Geometry check sheet. Reference: the model listing, model coordinates, mm. Face numbers are marked on the shaded views. A direction names the side the tool comes from. Coordinates: 2 decimals unless noted, no trailing zeros. Order: outer loops, then holes, each group sorted by start corner. A loop starts at its lowest first (then second) coordinate and runs counter-clockwise, first axis right, second up. Notation, with made-up numbers: (65, 19) - (86, 19) arc R12 cw to (86, 23) - close; hole circle Ø4 at (73, 37). An arc over 180 degrees is marked (long way). Put each result on its own line as item: value.
from build123d import *

# Parameters (mm, degrees)
SKETCH1_W           = 39.7
SKETCH1_H           = 39.7
BOSS_EXTRUDE1_DEPTH = 1
BOSS_EXTRUDE2_DEPTH = 13.6
SHELL1_START        = -12.6
SHELL1_DEPTH        = 13.6
SKETCH3_W           = 39.7
SKETCH3_H           = 39.7
SKETCH3_W_2         = 38.7
SKETCH3_H_2         = 38.7
CUT_EXTRUDE1_DEPTH  = 0.5
CUT_EXTRUDE2_REACH  = 33.642
SKETCH4_W           = 2
SKETCH4_H           = 0.3


# Read off the part's stored shape, not the designer's step: Shell1
with BuildPart() as part:
    # Sketch1 → Boss-Extrude1 (new body)
    with BuildSketch(Plane.XY):
        Rectangle(SKETCH1_W, SKETCH1_H)
    extrude(amount=BOSS_EXTRUDE1_DEPTH)

    # Sketch2 → Boss-Extrude2 (add)
    with BuildSketch(Plane(origin=(0, 0, 0), x_dir=(-1, 0, 0), z_dir=(0, 0, -1))):
        with BuildLine():
            Line((-8.3, -17.85), (8.3, -17.85))
            Line((8.3, -17.85), (8.3, -5.272366093))
            ThreePointArc((8.3, -5.272366093), (0, -0.85), (-8.3, -5.272366093))
            Line((-8.3, -5.272366093), (-8.3, -17.85))
        make_face()
    extrude(amount=BOSS_EXTRUDE2_DEPTH)

    # Shell1 outline → Shell1 (cut)
    with BuildSketch(Plane.XY.offset(SHELL1_START)):
        with BuildLine():
            Line((7.3, -16.85), (7.3, -5.585971125))
            ThreePointArc((7.3, -5.585971125), (0, -1.85), (-7.3, -5.585971125))
            Line((-7.3, -5.585971125), (-7.3, -16.85))
            Line((-7.3, -16.85), (7.3, -16.85))
        make_face()
    extrude(amount=SHELL1_DEPTH, mode=Mode.SUBTRACT)

    # Sketch3 → Cut-Extrude1 (cut)
    with BuildSketch(Plane.XY.offset(1)):
        Rectangle(SKETCH3_W, SKETCH3_H)
        Rectangle(SKETCH3_W_2, SKETCH3_H_2, mode=Mode.SUBTRACT)
    extrude(amount=-CUT_EXTRUDE1_DEPTH, mode=Mode.SUBTRACT)

    # Sketch4 → Cut-Extrude2 (cut, up to next)
    with BuildSketch(Plane(origin=(0, 0, -13.6), x_dir=(-1, 0, 0), z_dir=(0, 0, -1)), mode=Mode.PRIVATE) as cut_extrude2_sk1:
        with Locations((-5.5, -15.7)):
            Rectangle(SKETCH4_W, SKETCH4_H)
    cut_extrude2_tool1 = extrude(cut_extrude2_sk1.sketch, amount=-CUT_EXTRUDE2_REACH, mode=Mode.PRIVATE) & part.part
    # Sketch4 → Cut-Extrude2 (cut, up to next)
    with BuildSketch(Plane(origin=(0, 0, -13.6), x_dir=(-1, 0, 0), z_dir=(0, 0, -1)), mode=Mode.PRIVATE) as cut_extrude2_sk2:
        with Locations((5.5, -15.7)):
            Rectangle(SKETCH4_W, SKETCH4_H)
    cut_extrude2_tool2 = extrude(cut_extrude2_sk2.sketch, amount=-CUT_EXTRUDE2_REACH, mode=Mode.PRIVATE) & part.part
    add(cut_extrude2_tool1.solids().sort_by_distance((5.5, -15.7, -13.6))[0], mode=Mode.SUBTRACT)
    add(cut_extrude2_tool2.solids().sort_by_distance((-5.5, -15.7, -13.6))[0], mode=Mode.SUBTRACT)


solid = part.part
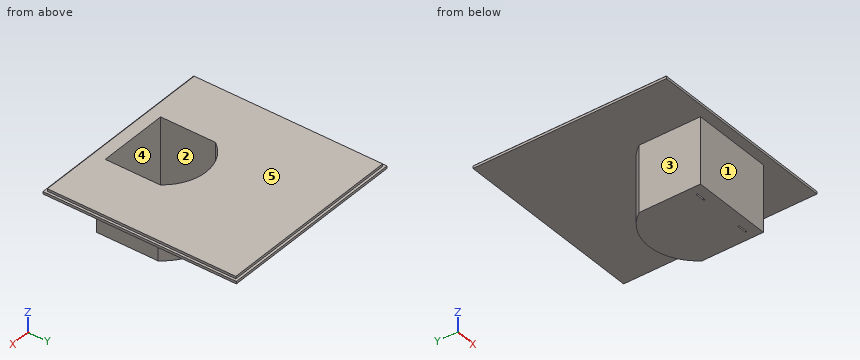
Q1. Section check A-A on z = -4.25. Record the boundary of the cut face in (x, y).
Answer block:
outline: (-8.3, -17.85) - (8.3, -17.85) - (8.3, -5.27) arc R10 ccw to (-8.3, -5.27) - close; hole (-7.3, -16.85) - (7.3, -16.85) - (7.3, -5.59) arc R9 ccw to (-7.3, -5.59) - close
Q2. Section check D-D on y = -4. Record the boundary of the cut face in (x, z).
Answer block:
outline: (-19.85, 0) - (-7.29, 0) - (-7.29, -13.6) - (7.29, -13.6) - (7.29, 0) - (19.85, 0) - (19.85, 0.5) - (19.35, 0.5) - (19.35, 1) - (5.84, 1) - (5.84, -12.6) - (-5.84, -12.6) - (-5.84, 1) - (-19.35, 1) - (-19.35, 0.5) - (-19.85, 0.5) - close
Q3. Depth check by flat-ended pin: pin 1 Ø1.1 at (x, z) = (5.5, -13) entering from -Y; pin 2 Ø1.1 at (x, z) = (-5, -13) entering from +Y; pin 3 Ø12 at (x, y) = (9.5, 2.5) entering from -Z. Enter the tip coordinate at first touch or a pass-through.
Answer block:
pin 1: stops at y = -17.85
pin 2: stops at y = -1.89
pin 3: stops at z = 0
Q4. Draft check along X on the marked faces 1, 2 and 3. Enter one of: pulls with the +X half, pulls with the -X half, needs draft (parallel to the pull), parting line crosses it, or undercut.
Answer block:
face 1: needs draft
face 2: undercut
face 3: pulls with the -X half
Q5. Thickness scan on L1, parallel to X at y = -7.5, z = -5.5; L2, parallel to Z at x = 11, y = -4; L3, parallel to Z at x = 1, y = -2.5. Record the ranges inside material, lowest first. Write a range as [from, to].
Answer block:
L1: x = [-8.3, -7.3], [7.3, 8.3]
L2: z = [0, 1]
L3: z = [-13.6, -12.6]
Q6. Section check B-B on x = -15. Record the boundary of the cut face in (y, z).
Answer block:
outline: (-19.85, 0) - (19.85, 0) - (19.85, 0.5) - (19.35, 0.5) - (19.35, 1) - (-19.35, 1) - (-19.35, 0.5) - (-19.85, 0.5) - close
Q7. Access from +Z, -Z, +X, -X, +Y, -Y to the whole of each face (thin tool, end or side, straight path). Record for the marked faces 4 and 5.
Answer block:
face 4: +Z
face 5: +Z, +X, -X, +Y, -Y
